from build123d import *

# Parameters (mm, degrees)
F0_R     = 1.3589
F1_DEPTH = 3.302
F2_R     = 1.13665
F3_DEPTH = 5.6388


with BuildPart() as f1:
    # F0 (on Right) → F1 (new body)
    with BuildSketch(Plane.YZ):
        Circle(F0_R)
    extrude(amount=F1_DEPTH)

    # F2 (on face) → F3 (join)
    with BuildSketch(Plane(origin=(0, 0, 0), x_dir=(0, -1, 0), z_dir=(-1, 0, 0))):
        Circle(F2_R)
    extrude(amount=F3_DEPTH)

    # F4 (on Top) → F5 (revolve)
    with BuildSketch(Plane.XY):
        with BuildLine():
            Line((-6.7818, 0), (-5.6388, 0))
            Line((-5.6388, 0), (-5.6388, 1.13665))
            ThreePointArc((-5.6388, 1.13665), (-6.446636, 0.805981), (-6.7818, 0))
        make_face()
    revolve(axis=Axis((-6.2103, 0, 0), (-1, 0, 0)))

    # F6 (on Top) → F7 (revolve)
    with BuildSketch(Plane.XY):
        with BuildLine():
            Line((6.0452, 0), (3.302, 0))
            Line((3.302, 0), (3.302, -1.3589))
            ThreePointArc((3.302, -1.3589), (3.737246, -0.768925), (4.468674, -0.81915))
            Line((4.468674, -0.81915), (5.333006, -0.81915))
            Line((5.333006, -0.81915), (6.0452, -0.407965))
            Line((6.0452, -0.407965), (6.0452, 0))
        make_face()
    revolve(axis=Axis((4.6736, 0, 0), (-1, 0, 0)))


solid = f1.part
Can you work these out from the model? Positions are in its coordinate system, mm. A direction names the side the tool comes from. Give positions to 0.01 mm unless a question says otherwise; leave off trailing zeros. Order: outer loops, then holes, each group sorted by start corner. A loop starts at its lowest first (then second) coordinate and runs counter-clockwise, first axis right, second up. Notation, with made-up numbers: M -28.5,-29 L 4.5,-29 A22 ccw 4.5,7 Z; hole C -13,-39.75 d3. An arc over 180 degrees is marked long. Use a Markdown table: item, result. Add a question column.
Item 1: If I drill on L1, parallel to Z at x = -2.75, y = -0.05; L2, parallel to Z at x = 1.25, y = 0.45; L3, parallel to X at y = 0.7, z = -0.55, over which ranges is the centre line in solid material (lowest first)? Write a range as [from, to].
Item 2: Suppose I cut it at B-B (x = 0.25). List the corners of the cut face in (y, z) for me.
Item 3: For faces 1 (the cylindrical face through (4.907, 0.604, 0.554)), 2 (the cylindrical face through (1.6, 1.3, 0.4)), 3 (the cylindrical face through (-2.78, 0.838, 0.768)), which set-ups out of +Z, -Z, +X, -X, +Y, -Y let a thin tool reach every point of the face, with its end or its side?
Item 4: Suppose I cut it at A-A (x = 5). List the corners of the cut face in (y, z) for me, then the cut area to 3 significant figures.
Item 5: Will these pins go through, and if not, where does the flat tip stop? pin 1 (1 mm diameter, centred on x = 4.5, z = 0, fed in from -Y); pin 2 (1 mm diameter, centred on x = -2, y = -1, fed in from +Z); pin 3 (0.8 mm diameter, centred on y = 0, z = 0.5, fed in from -X).
Answer sheet:
| question | item | result |
|---|---|---|
| 1 | L1 | z = [-1.14, 1.14] |
| 1 | L2 | z = [-1.28, 1.28] |
| 1 | L3 | x = [-6.35, 3.55] |
| 2 | outline | C 0,0 d2.72 |
| 3 | face 1 | +X |
| 3 | face 2 | +X, -X |
| 3 | face 3 | -X |
| 4 | outline | C 0,0 d1.64 |
| 4 | area | 2.11 mm² |
| 5 | pin 1 | stops at y = -0.82 |
| 5 | pin 2 | stops at z = 1.02 |
| 5 | pin 3 | stops at x = -6.78 |
